Answer from the drawing. Dimensions are ordinates in mm from the lowest x, y and z of the part. Coordinates: 2 decimals unless noted, no trailing zeros. Loops run counter-clockwise (first coordinate to the right, second up) from the corner with the lowest first, then second, coordinate; pieces in that order, holes last. Notation, with made-up numbers: (69.25, -20.75) - (78.25, -20.75) arc R8 ccw to (78.25, -15.75) - close; hole circle Ø9 at (89, 5.25). An arc over 180 degrees is marked (long way). Use one line per item in the form item = value. Start each with the question number.
1) A cutting plane is placed at A-A (x = 57). Give the vertices of the cut face in (y, z), and give its area (3 significant figures).
2) A cutting plane is placed at D-D (z = 6.5). Give the vertices of the cut face in (x, y), and give its area (3 significant figures).
3) A cutting plane is placed at B-B (z = 10). Give the vertices of the cut face in (x, y).
4) A cutting plane is placed at C-C (y = 1). Give the vertices of the cut face in (x, z).
5) Consider line 1 (X direction, y = 3.5, z = 10); line 2 (Z direction, x = 57, y = 5.75); line 3 (X direction, y = 4.5, z = 11.25). Determine where each line is inside the solid, lowest interval first.
6) Each of these flat-tipped pins is pushed along its axis until it touches: P1, Ø1, axis at y = 6.5, z = 12, coming from the -X side; P2, Ø1.3, axis at x = 45, z = 6, coming from the -Y side. Where does it stop, or does it pass through?
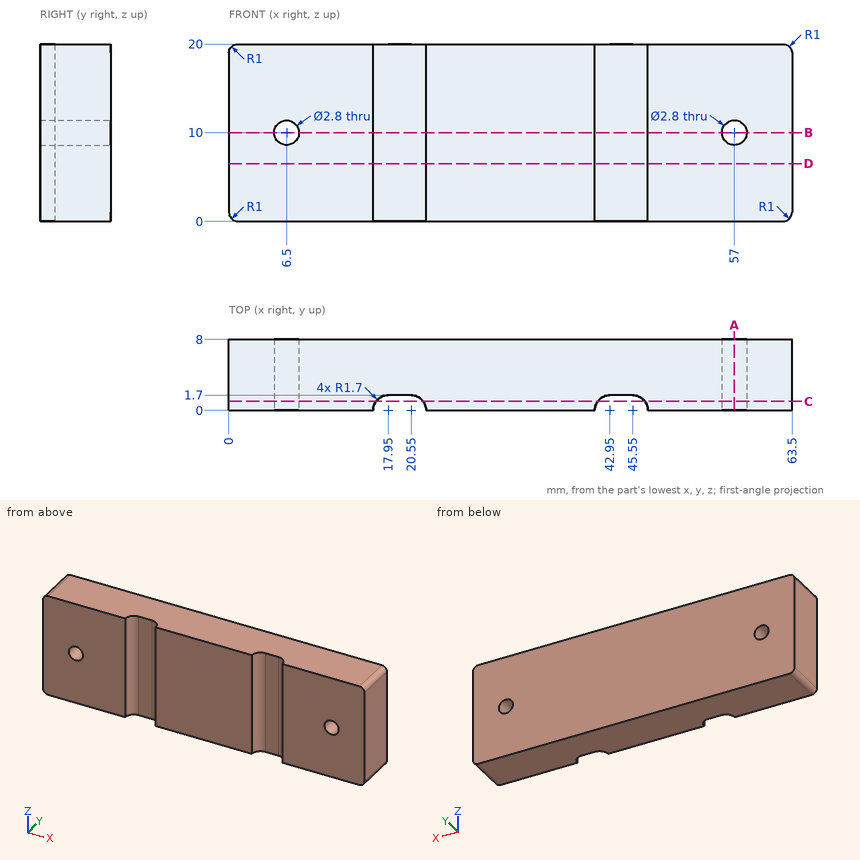
Found:
q1.outline = (0, 0) - (8, 0) - (8, 8.6) - (0, 8.6) - close; (0, 11.4) - (8, 11.4) - (8, 20) - (0, 20) - close
q1.area = 138 mm^2
q2.outline = (0, 0) - (16.25, 0) arc R1.7 cw to (17.95, 1.7) - (20.55, 1.7) arc R1.7 cw to (22.25, 0) - (41.25, 0) arc R1.7 cw to (42.95, 1.7) - (45.55, 1.7) arc R1.7 cw to (47.25, 0) - (63.5, 0) - (63.5, 8) - (0, 8) - close
q2.area = 490 mm^2
q3.outline = (0, 0) - (5.1, 0) - (5.1, 8) - (0, 8) - close; (7.9, 0) - (16.25, 0) arc R1.7 cw to (17.95, 1.7) - (20.55, 1.7) arc R1.7 cw to (22.25, 0) - (41.25, 0) arc R1.7 cw to (42.95, 1.7) - (45.55, 1.7) arc R1.7 cw to (47.25, 0) - (55.6, 0) - (55.6, 8) - (7.9, 8) - close; (58.4, 0) - (63.5, 0) - (63.5, 8) - (58.4, 8) - close
q4.outline = (0, 1) arc R1 ccw to (1, 0) - (16.58, 0) - (16.58, 20) - (1, 20) arc R1 ccw to (0, 19) - close; (21.92, 0) - (41.58, 0) - (41.58, 20) - (21.92, 20) - close; (46.92, 0) - (62.5, 0) arc R1 ccw to (63.5, 1) - (63.5, 19) arc R1 ccw to (62.5, 20) - (46.92, 20) - close; hole circle Ø2.8 at (6.5, 10); hole circle Ø2.8 at (57, 10)
q5.line_1 = 0 to 5.1, 7.9 to 55.6, 58.4 to 63.5
q5.line_2 = 0 to 8.6, 11.4 to 20
q5.line_3 = 0 to 5.87, 7.13 to 56.37, 57.63 to 63.5
q6.P1 = 0
q6.P2 = 1.7
